Can you work these out from the drawing? Everything is in mm from the part's minimum corner. Round coordinates to 2 decimals unless told otherwise and drop trailing zeros. Loops run counter-clockwise (first coordinate to the right, second up) from the corner with the lowest first, then second, coordinate; pieces in that order, holes last. Notation, with made-up numbers: M 46,63.25 L 73,63.25 A21 cw 73,101.25 Z; hole C 27,26 d6. An arc over 180 degrees is marked long. Answer in a Markdown table with one row per item.
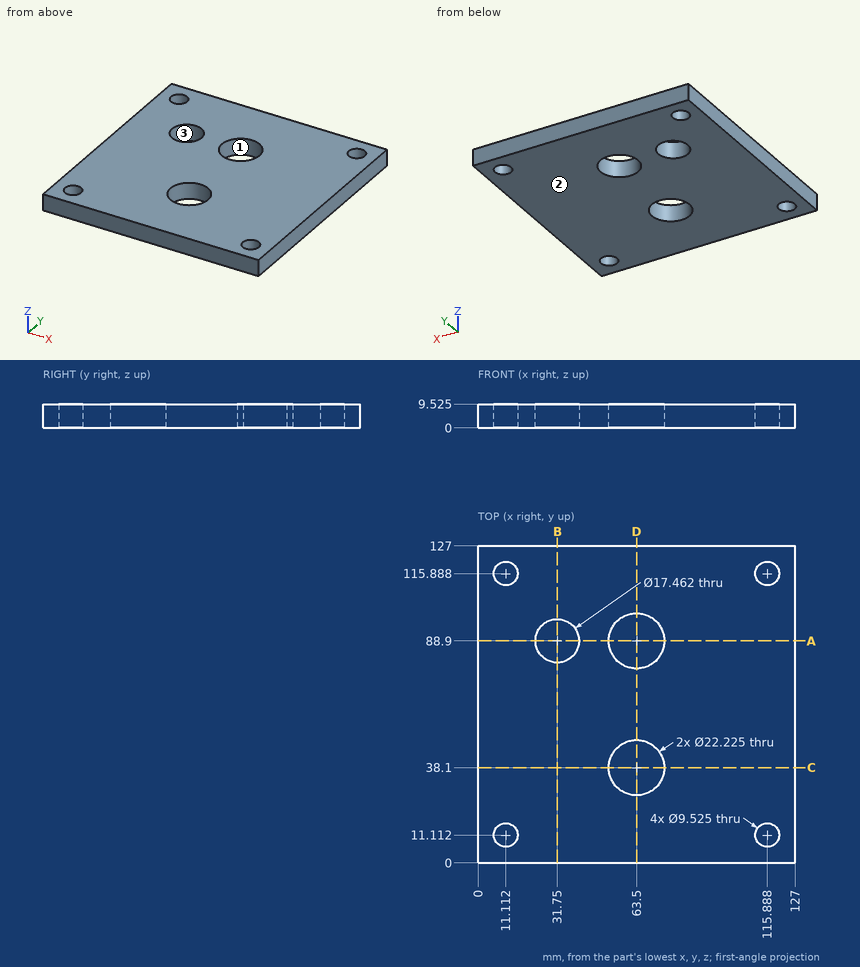
1) I want a section at D-D, the plane x = 63.5. Please give me the cut outline in (y, z) (1 decimal).
Computed:
| item | result |
|---|---|
| outline | M 0,0 L 27,0 L 27,9.5 L 0,9.5 Z; M 49.2,0 L 77.8,0 L 77.8,9.5 L 49.2,9.5 Z; M 100,0 L 127,0 L 127,9.5 L 100,9.5 Z |
2) I need wall thicknesses on line 1 (Y direction, x = 63.5, z = 4.25); line 2 (Y direction, x = 31.75, z = 4.5); line 3 (Y direction, x = 58, z = 7) (1 decimal). Which ranges of each line are inside material? Lowest first, please.
Computed:
| item | result |
|---|---|
| line 1 | y = 0 to 26.99, 49.21 to 77.79, 100.01 to 127 |
| line 2 | y = 0 to 80.17, 97.63 to 127 |
| line 3 | y = 0 to 28.4, 47.8 to 79.2, 98.6 to 127 |
3) I want a section at B-B, the plane x = 31.75. Please give me the cut outline in (y, z) (1 decimal), plus the area to 3 significant figures.
Computed:
| item | result |
|---|---|
| outline | M 0,0 L 80.2,0 L 80.2,9.5 L 0,9.5 Z; M 97.6,0 L 127,0 L 127,9.5 L 97.6,9.5 Z |
| area | 1,040 mm² |
4) If we mould it in two halves opening along Y, with no side actions, what happens to the marked faces 1, 2 and 3? For each: released by +Y, released by -Y, zero draft, split by the parting line, or undercut.
Computed:
| item | result |
|---|---|
| face 1 | undercut |
| face 2 | zero draft |
| face 3 | undercut |
5) I want a section at A-A, the plane y = 88.9. Please give me the cut outline in (x, z) (1 decimal).
Computed:
| item | result |
|---|---|
| outline | M 0,0 L 23,0 L 23,9.5 L 0,9.5 Z; M 40.5,0 L 52.4,0 L 52.4,9.5 L 40.5,9.5 Z; M 74.6,0 L 127,0 L 127,9.5 L 74.6,9.5 Z |
6) I want a section at C-C, the plane y = 38.1. Please give me the cut outline in (x, z) (1 decimal), plus the area to 3 significant figures.
Computed:
| item | result |
|---|---|
| outline | M 0,0 L 52.4,0 L 52.4,9.5 L 0,9.5 Z; M 74.6,0 L 127,0 L 127,9.5 L 74.6,9.5 Z |
| area | 998 mm² |
